Model file for the job. Use its own axes, mm. Face numbers are marked on the shaded views. A direction names the side the tool comes from. Coordinates: 2 decimals unless noted, no trailing zeros. Order: outer loops, then holes, each group sorted by start corner. A loop starts at its lowest first (then second) coordinate and runs counter-clockwise, first axis right, second up.
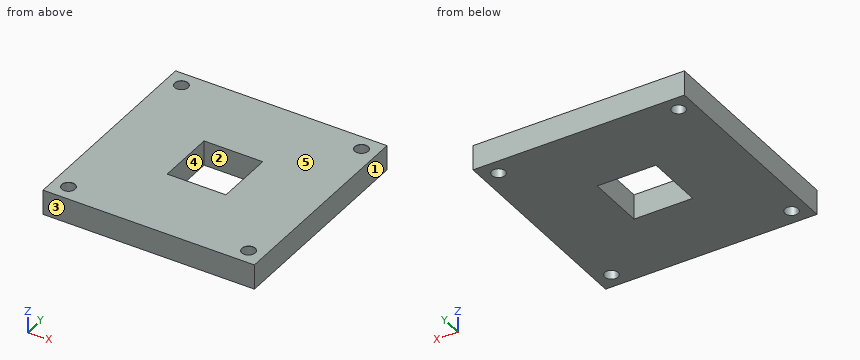
from build123d import *

# Parameters (mm, degrees)
SKETCH1_W           = 54
SKETCH1_H           = 54
BOSS_EXTRUDE1_DEPTH = 6.35
SKETCH6_W           = 15
SKETCH6_H           = 15
CUT_EXTRUDE1_DEPTH  = 10


# Read off the part's stored shape, not the designer's step: M3 Clearance Hole1
with BuildPart() as part:
    # Sketch1 → Boss-Extrude1 (new body)
    with BuildSketch(Plane.XY):
        Rectangle(SKETCH1_W, SKETCH1_H)
    extrude(amount=-BOSS_EXTRUDE1_DEPTH)

    # M3 Clearance Hole1 outline → M3 Clearance Hole1 (revolve, cut)
    with BuildSketch(Plane(origin=(23, -23, 0), x_dir=(1, 0, 0), z_dir=(0, -1, 0))):
        Polygon((0, -6.35), (1.7, -6.35), (1.7, -0.04330127), (1.725, 0), (0, 0), align=None)
    revolve(axis=Axis((23, -23, 0), (0, 0, 1)), mode=Mode.SUBTRACT)

    # M3 Clearance Hole1 2 outline → M3 Clearance Hole1 2 (revolve, cut)
    with BuildSketch(Plane(origin=(-23, 23, 0), x_dir=(1, 0, 0), z_dir=(0, -1, 0))):
        Polygon((0, -6.35), (1.7, -6.35), (1.7, -0.04330127), (1.725, 0), (0, 0), align=None)
    revolve(axis=Axis((-23, 23, 0), (0, 0, 1)), mode=Mode.SUBTRACT)

    # M3 Clearance Hole1 3 outline → M3 Clearance Hole1 3 (revolve, cut)
    with BuildSketch(Plane(origin=(-23, -23, 0), x_dir=(1, 0, 0), z_dir=(0, -1, 0))):
        Polygon((0, -6.35), (1.7, -6.35), (1.7, -0.04330127), (1.725, 0), (0, 0), align=None)
    revolve(axis=Axis((-23, -23, 0), (0, 0, 1)), mode=Mode.SUBTRACT)

    # M3 Clearance Hole1 4 outline → M3 Clearance Hole1 4 (revolve, cut)
    with BuildSketch(Plane(origin=(23, 23, 0), x_dir=(1, 0, 0), z_dir=(0, -1, 0))):
        Polygon((0, -6.35), (1.7, -6.35), (1.7, -0.04330127), (1.725, 0), (0, 0), align=None)
    revolve(axis=Axis((23, 23, 0), (0, 0, 1)), mode=Mode.SUBTRACT)

    # Sketch6 → Cut-Extrude1 (cut)
    with BuildSketch(Plane.XY):
        Rectangle(SKETCH6_W, SKETCH6_H)
    extrude(amount=-CUT_EXTRUDE1_DEPTH, mode=Mode.SUBTRACT)


solid = part.part
Q1. Cut at C-C, the plane z = -2.25. List the corners of the cut face in (x, y).
Established:
outline: (-27, -27) - (27, -27) - (27, 27) - (-27, 27) - close; hole circle Ø3.4 at (-23, -23); hole circle Ø3.4 at (-23, 23); hole (-7.5, -7.5) - (7.5, -7.5) - (7.5, 7.5) - (-7.5, 7.5) - close; hole circle Ø3.4 at (23, -23); hole circle Ø3.4 at (23, 23)
Q2. Cut at A-A, the plane y = -23. List the corners of the cut face in (x, z) (3 decimals).
Established:
outline: (-27, -6.35) - (-24.7, -6.35) - (-24.7, -0.043) - (-24.725, 0) - (-27, 0) - close; (-21.3, -6.35) - (21.3, -6.35) - (21.3, -0.043) - (21.275, 0) - (-21.275, 0) - (-21.3, -0.043) - close; (24.7, -6.35) - (27, -6.35) - (27, 0) - (24.725, 0) - (24.7, -0.043) - close
Q3. Probe line 1 (Y direction, x = -23, z = -3.5); line 2 (Y direction, x = -3, z = -4). List the from-to ranges inside material, lowest first.
Established:
line 1: y = -27 to -24.7, -21.3 to 21.3, 24.7 to 27
line 2: y = -27 to -7.5, 7.5 to 27
Q4. Which spindle directions (+Z, -Z, +X, -X, +Y, -Y) get a long thin tool onto all of the face, cutting with end or side? Do the marked faces 1 and 2. Say none if no direction does.
Established:
face 1: +Z, -Z, +X, +Y, -Y
face 2: +Z, -Z
Q5. Mould opens along Y. For the marked faces 3, 4 and 5 say: pulls with the +Y half, pulls with the -Y half, needs draft (parallel to the pull), parting line crosses it, or undercut.
Established:
face 3: pulls with the -Y half
face 4: undercut
face 5: needs draft
Q6. Cut at D-D, the plane y = -0.5. List the corners of the cut face in (x, z).
Established:
outline: (-27, -6.35) - (-7.5, -6.35) - (-7.5, 0) - (-27, 0) - close; (7.5, -6.35) - (27, -6.35) - (27, 0) - (7.5, 0) - close
